from build123d import *

# Parameters (mm, degrees)
F0_W      = 72
F0_H      = 102
F1_DEPTH  = 25
F3_DEPTH  = 23
F4_W      = 9.5
F4_H      = 4.5
F4_R      = 3.5
F5_DEPTH  = 3
F6_DEPTH  = 3
F7_W      = 8
F7_H      = 4
F8_DEPTH  = 3
F10_W     = 23
F10_H     = 74
F10_W_2   = 19
F10_H_2   = 70
F11_DEPTH = 18
F12_W     = 2
F12_H     = 6.944833
F13_DEPTH = 16
F14_R     = 2.5
F15_DEPTH = 75
F17_DEPTH = 6
F18_SIZE  = 2.5


with BuildPart() as f1:
    # F0 (on Top) → F1 (new body)
    with BuildSketch(Plane.XY):
        Rectangle(F0_W, F0_H)
    extrude(amount=F1_DEPTH)

    # F2 (on face) → F3 (cut)
    with BuildSketch(Plane.XY.offset(25)):
        Polygon((34, 42.058192), (27.058192, 49), (-27.058192, 49), (-34, 42.058192), (-34, -42.058192), (-27.058192, -49), (34, -49), align=None)
    extrude(amount=-F3_DEPTH, mode=Mode.SUBTRACT)

    # F4 (on face) → F5 (cut)
    with BuildSketch(Plane.XZ.offset(51)):
        with Locations((26.25, 9.523708)):
            Rectangle(F4_W, F4_H)
        with Locations((11.4543, 10.823708)):
            Circle(F4_R)
    extrude(amount=-F5_DEPTH, mode=Mode.SUBTRACT)

    # F4 (on face) → F6 (cut)
    with BuildSketch(Plane.XZ.offset(51)):
        with Locations((26.25, 9.523708)):
            Rectangle(F4_W, F4_H)
        with Locations((11.4543, 10.823708)):
            Circle(F4_R)
    extrude(amount=-F6_DEPTH, mode=Mode.SUBTRACT)

    # F7 (on face) → F8 (cut)
    with BuildSketch(Plane.YZ.offset(36)):
        with Locations((-36, 9.25)):
            Rectangle(F7_W, F7_H)
    extrude(amount=-F8_DEPTH, mode=Mode.SUBTRACT)

    # F10 (on face) → F11 (join)
    with BuildSketch(Plane.XY.offset(2)):
        with Locations((-18.5, -1)):
            Rectangle(F10_W, F10_H)
        with Locations((-18.5, -1)):
            Rectangle(F10_W_2, F10_H_2, mode=Mode.SUBTRACT)
    extrude(amount=F11_DEPTH)

    # F12 (on face) → F13 (cut)
    with BuildSketch(Plane.XY.offset(20)):
        with Locations((-29, -32.527583)):
            Rectangle(F12_W, F12_H)
        with Locations((-8, -32.527583)):
            Rectangle(F12_W, F12_H)
    extrude(amount=-F13_DEPTH, mode=Mode.SUBTRACT)

    # F14 (on face) → F15 (cut)
    with BuildSketch(Plane.XZ.offset(38)):
        with Locations((-18.5, 11)):
            Circle(F14_R)
    extrude(amount=-F15_DEPTH, mode=Mode.SUBTRACT)

    # F16 (on face) → F17 (join)
    with BuildSketch(Plane.XY.offset(25)):
        Polygon((34, -41.767824), (26.534403, -49), (34, -49), align=None)
    extrude(amount=-F17_DEPTH)

    # F18
    f18_edges = [f1.edges().sort_by_distance(p)[0] for p in [
        (30.267201, -45.383912, 19),
    ]]
    chamfer(f18_edges, length=F18_SIZE)


solid = f1.part
Verification items for the finished model (mm, model axes). A direction names the side the tool comes from. Round coordinates to 2 decimals unless told otherwise and drop trailing zeros. Loops run counter-clockwise (first coordinate to the right, second up) from the corner with the lowest first, then second, coordinate; pieces in that order, holes last. Notation, with made-up numbers: M 8.25,31.25 L 32.25,31.25 A23 ccw 32.25,70.25 Z; hole C 72.5,-14 d10. An arc over 180 degrees is marked long. Write each question's results on one line, items separated by ' | '.
1) Section check C-C on y = -34. Record the boundary of the cut face in (x, z).
Checks:
outline: M -36,0 L 36,0 L 36,7.25 L 34,7.25 L 34,2 L -7,2 L -7,4 L -9,4 L -9,2 L -28,2 L -28,4 L -30,4 L -30,2 L -34,2 L -34,25 L -36,25 Z; M 34,11.25 L 36,11.25 L 36,25 L 34,25 Z
2) Mould release check, pull along Y, two halves, no side actions. Record for faces 5 (the cylindrical face through (14.687, -50.014, 9.483)), 6 (the flat face through (-21, -36, 13)), 7 (the flat face through (-1, -51, 12)): released by +Y, released by -Y, zero draft, split by the parting line, or undercut.
Checks:
face 5: zero draft | face 6: undercut | face 7: released by -Y
3) Access from +Z, -Z, +X, -X, +Y, -Y to the whole of each face (thin tool, end or side, straight path). Record for faces 1 (the flat face through (26, -50, 7.274)), 2 (the flat face through (-36, -1, 12)), 3 (the flat face through (35, -32, 9)), 4 (the flat face through (-21, 34, 13)).
Checks:
face 1: -Y | face 2: +Z, -Z, -X, +Y, -Y | face 3: +X | face 4: +Z
4) Section check D-D on x = -1.5. Record the boundary of the cut face in (y, z), then the cut area to 3 significant figures.
Checks:
outline: M -51,0 L 51,0 L 51,25 L 49,25 L 49,2 L -49,2 L -49,25 L -51,25 Z | area: 296 mm2
5) Section check A-A on z = 17.25. Record the boundary of the cut face in (x, y), then the cut area to 3 significant figures.
Checks:
outline: M -36,-51 L 36,-51 L 36,51 L -36,51 Z; M -30,-38 L -7,-38 L -7,-36 L -30,-36 Z; M -30,-29.06 L -28,-29.06 L -28,34 L -9,34 L -9,-29.06 L -7,-29.06 L -7,36 L -30,36 Z; hole M -34,-42.06 L -27.06,-49 L 34,-49 L 34,42.06 L 27.06,49 L -27.06,49 L -34,42.06 Z | area: 1,100 mm2
6) Gauge pin test, flat ends, axial feed: P1, Ø20.5, axis at x = -16, y = -21, coming from the +Z side; P2, Ø6, axis at x = 24.5, z = 8, coming from the -Y side; P3, Ø2, axis at x = -14, y = 10.5, coming from the +Z side; P4, Ø1, axis at x = -29, y = -33.5, coming from the +Z side. Record the tip position at first contact, or that the pin passes through.
Checks:
P1: stops at z = 20 | P2: stops at y = -51 | P3: stops at z = 2 | P4: stops at z = 4
7) Section check B-B on x = -18.5. Record the boundary of the cut face in (y, z).
Checks:
outline: M -51,0 L 51,0 L 51,25 L 49,25 L 49,2 L 36,2 L 36,8.5 L 34,8.5 L 34,2 L -36,2 L -36,8.5 L -38,8.5 L -38,2 L -49,2 L -49,25 L -51,25 Z; M -38,13.5 L -36,13.5 L -36,20 L -38,20 Z; M 34,13.5 L 36,13.5 L 36,20 L 34,20 Z
8) Scan lines: L1, parallel to X at y = -2, z = 19.5; L2, parallel to Y at x = -23, z = 17; L3, parallel to X at y = -37, z = 3.25. Record each from-to range of solid material in increasing order. Write a range as from..to.
Checks:
L1: x = -36..-34, -30..-28, -9..-7, 34..36 | L2: y = -51..-49, -38..-36, 34..36, 49..51 | L3: x = -36..-34, -30..-7, 34..36
